from build123d import *

# Parameters (mm, degrees)
F1_DEPTH = 50
F2_DEPTH = 4
F3_R     = 4.25
F4_DEPTH = 25
F5_R     = 4.25
F6_DEPTH = 25
F7_R     = 5


with BuildPart() as f1:
    # F0 (on Top) → F1 (new body)
    with BuildSketch(Plane.XY):
        Polygon((-14.747666, -4.400732), (-9.747666, -4.400732), (-9.747666, 25.599268), (15.252334, 25.599268), (15.252334, 30.599268), (-14.747666, 30.599268), align=None)
    extrude(amount=F1_DEPTH)

    # F0 (on Top) → F2 (join)
    with BuildSketch(Plane.XY):
        Polygon((-9.747666, 25.599268), (-9.747666, -4.400732), (15.252334, 25.599268), align=None)
    extrude(amount=F2_DEPTH)

    # F3 (on face) → F4 (cut)
    with BuildSketch(Plane(origin=(-14.747666, 0, 0), x_dir=(0, -1, 0), z_dir=(-1, 0, 0))):
        with Locations((-4.599268, 17.855786)):
            Circle(F3_R)
        with BuildLine():
            ThreePointArc((-0.349268, 45), (-4.599268, 49.25), (-8.849268, 45))
            ThreePointArc((-8.849268, 45), (-4.599268, 40.75), (-0.349268, 45))
        make_face()
        with BuildLine():
            Line((-0.349268, 50), (-8.849268, 50))
            Line((-8.849268, 50), (-8.849268, 45))
            ThreePointArc((-8.849268, 45), (-4.599268, 49.25), (-0.349268, 45))
            Line((-0.349268, 45), (-0.349268, 50))
        make_face()
    extrude(amount=-F4_DEPTH, mode=Mode.SUBTRACT)

    # F5 (on face) → F6 (cut)
    with BuildSketch(Plane(origin=(0, 30.599268, 0), x_dir=(-1, 0, 0), z_dir=(0, 1, 0))):
        with Locations((-0.252334, 34.25)):
            Circle(F5_R)
        with Locations((-0.252334, 10.25)):
            Circle(F5_R)
    extrude(amount=-F6_DEPTH, mode=Mode.SUBTRACT)

    # F7
    f7_edges = [f1.edges().sort_by_distance(p)[0] for p in [
        (-9.747666, 25.599268, 27),
    ]]
    fillet(f7_edges, radius=F7_R)


solid = f1.part
Here's how the part is built. I have some questions about the finished solid (model axes, mm). A direction names the side the tool comes from. Coordinates: 2 decimals unless noted, no trailing zeros. Loops run counter-clockwise (first coordinate to the right, second up) from the corner with the lowest first, then second, coordinate; pieces in that order, holes last. Notation, with made-up numbers: (8.5, 61) -> (66.5, 61) arc R18 cw to (66.5, 90) -> close; hole circle Ø7 at (69, 51). An arc over 180 degrees is marked (long way). Use one line per item in the form item = value. Start each with the question number.
(1) If we section it at C-C (x = -2.5): Please give me the cut outline in (y, z).
(2) Will these pins go through, and if not, where does the flat tip stop? pin 1 (3 mm diameter, centred on x = -1.5, y = 14, fed in from +Z); pin 2 (12.5 mm diameter, centred on y = 11.5, z = 30.5, fed in from +X); pin 3 (5 mm diameter, centred on x = 7.5, y = 20.5, fed in from -Z); pin 4 (1.5 mm diameter, centred on x = -0.5, z = 44.5, fed in from -Y).
(3) On a 3-axis mill with a long thin cutter (end or side, diameter ignored), from which of +Z, -Z, +X, -X, +Y, -Y can I reach the whole of each face in a straight line? I mean faces 1 (the face through (0, 30.599, 25)), 2 (the face through (-9.748, 8, 27)), 3 (the face through (-12, 8.849, 48)). Say none if no direction works.
(4) We'd pull the mould along X, two halves only. Please class faces 4 (the face through (-8.32, 24.1, 27.32)), 5 (the face through (1.17, 28.13, 6.1)), 6 (the face through (-7, 27, 50)): pulls with the +X half, pulls with the -X half, needs draft (parallel to the pull), parting line crosses it, or undercut.
(5) If we section it at B-B (y = 2.5): Please give me the cut outline in (x, z).
(6) If we section it at A-A (z = 10.25): Please give me the cut outline in (x, y), then the cut area to 3 significant figures.
(7) If we section it at D-D (z = 16.5): Please give me the cut outline in (x, y).
(8) Please list where these lines run through material, in increasing order: line 1 along X through (y, z) = (28, 10); line 2 along X through (y, z) = (15.5, 5); line 3 along Y through (x, z) = (10.25, 19).
Verdict:
q1.outline = (4.3, 0) -> (30.6, 0) -> (30.6, 7.01) -> (25.6, 7.01) -> (25.6, 4) -> (4.3, 4) -> close; (25.6, 13.49) -> (30.6, 13.49) -> (30.6, 31.01) -> (25.6, 31.01) -> close; (25.6, 37.49) -> (30.6, 37.49) -> (30.6, 50) -> (25.6, 50) -> close
q2.pin_1 = 4
q2.pin_2 = -9.75
q2.pin_3 = 0
q2.pin_4 = 25.6
q3.face_1 = +Z, -Z, +X, -X, +Y
q3.face_2 = +Z, +X, -Y
q3.face_3 = +Z, +X, -X
q4.face_4 = pulls with the +X half
q4.face_5 = undercut
q4.face_6 = needs draft
q5.outline = (-14.75, 0) -> (-4, 0) -> (-4, 4) -> (-9.75, 4) -> (-9.75, 14.16) -> (-14.75, 14.16) -> close; (-14.75, 21.55) -> (-9.75, 21.55) -> (-9.75, 41.3) -> (-14.75, 41.3) -> close
q6.outline = (-14.75, -4.4) -> (-9.75, -4.4) -> (-9.75, 20.6) arc R5 cw to (-4.75, 25.6) -> (-4, 25.6) -> (-4, 30.6) -> (-14.75, 30.6) -> close; (4.5, 25.6) -> (15.25, 25.6) -> (15.25, 30.6) -> (4.5, 30.6) -> close
q6.area = 263 mm²
q7.outline = (-14.75, -4.4) -> (-9.75, -4.4) -> (-9.75, 0.57) -> (-14.75, 0.57) -> close; (-14.75, 8.63) -> (-9.75, 8.63) -> (-9.75, 20.6) arc R5 cw to (-4.75, 25.6) -> (15.25, 25.6) -> (15.25, 30.6) -> (-14.75, 30.6) -> close
q8.line_1 = -14.75 to -3.99, 4.49 to 15.25
q8.line_2 = -14.75 to -9.75
q8.line_3 = 25.6 to 30.6
